Geometry: final body of the model. Coordinates: model frame, mm. Face numbers are marked on the shaded views. A direction names the side the tool comes from. Give positions to 0.01 mm unless a question says otherwise; leave off trailing zeros. Order: outer loops, then holes, each group sorted by start corner. A loop starts at its lowest first (then second) coordinate and runs counter-clockwise, first axis right, second up. Notation, with made-up numbers: (57, -13) - (112, -13) arc R29 ccw to (112, 11) - close; hole circle Ø6 at (62, -8). An arc over 180 degrees is marked (long way). Put each result on its own line as item: value. Start each with the question number.
1. Section B-B on x = -45. Return the cut outline in (y, z).
2. Section D-D on y = 6.25. Return the cut outline in (x, z).
3. Ray query, line 1 along X through (y, z) = (16.5, 3); line 2 along Z through (x, y) = (-31.5, 14.75); line 3 along X through (y, z) = (3, 25). Return the intervals inside material, ascending. Write a range as from..to.
4. First-contact query: P1, Ø15, axis at x = -91.313, y = 14.351, coming from the +Z side. Flat tip, straight axial feed; report the tip coordinate or a pass-through.
5. Set-up query: the marked faces 1 and 2. Return all of +Z, -Z, +X, -X, +Y, -Y with unobstructed straight access to the full face (end or side cutting, diameter ignored); none if empty.
6. Section C-C on y = 18. Return the cut outline in (x, z).
7. Mould query, pull axis Z, two halves, no side actions, for the marked faces 3, 4, 5 and 6. Classes: pulls with the +Z half, pulls with the -Z half, needs draft (parallel to the pull), parting line crosses it, or undercut.
8. Section A-A on z = 23.5. Return the cut outline in (x, y).
from build123d import *

# Parameters (mm, degrees)
EXTRUDE1_DEPTH = 28.702
SKETCH2_R      = 11.303
EXTRUDE2_DEPTH = 93.609737566
SKETCH3_R      = 6.35
EXTRUDE3_DEPTH = 12.7
SKETCH4_R      = 4.7625
EXTRUDE4_DEPTH = 117.756868277


with BuildPart() as part:
    # Sketch1 → Extrude1 (new body)
    with BuildSketch(Plane(origin=(0, 0, 0), x_dir=(1, 0, 0), z_dir=(0, 1, 0))):
        Polygon((0, 0), (0, -35.052), (-28.702, -35.052), (-28.702, -6.35), (-109.474, -6.35), (-109.474, 0), align=None)
    extrude(amount=EXTRUDE1_DEPTH)

    # Sketch2 → Extrude2 (cut, through all)
    with BuildSketch(Plane.ZY.offset(28.702)):
        with Locations((20.701, 14.351)):
            Circle(SKETCH2_R)
    extrude(amount=-EXTRUDE2_DEPTH, mode=Mode.SUBTRACT)

    # Sketch3 → Extrude3 (cut)
    with BuildSketch(Plane.XY.offset(35.052)):
        with Locations((-14.351, 14.351)):
            Circle(SKETCH3_R)
    extrude(amount=-EXTRUDE3_DEPTH, mode=Mode.SUBTRACT)

    # Sketch4 → Extrude4 (cut, through all)
    with BuildSketch(Plane.XY.offset(6.35)):
        with Locations((-91.313, 14.351)):
            Circle(SKETCH4_R)
        with Locations(Location((-46.863, 14.351, 0), (0, 0, 180))):
            Circle(SKETCH4_R)
    extrude(amount=-EXTRUDE4_DEPTH, mode=Mode.SUBTRACT)


solid = part.part
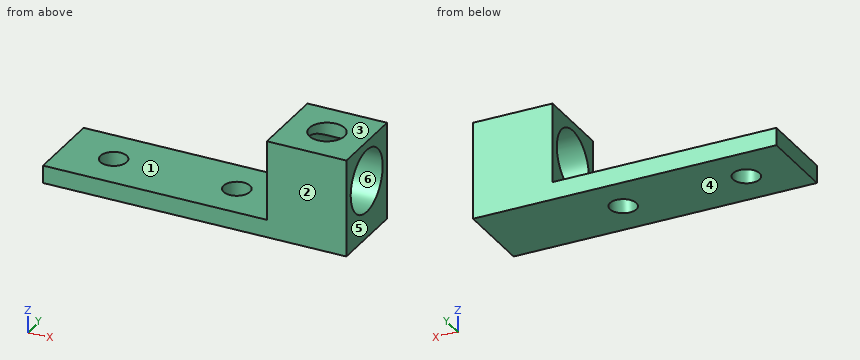
Resolved:
1. outline: (0, 0) - (9.97, 0) - (9.97, 6.35) - (0, 6.35) - close; (18.73, 0) - (28.7, 0) - (28.7, 6.35) - (18.73, 6.35) - close
2. outline: (-109.47, 0) - (0, 0) - (0, 12.82) - (-28.7, 12.82) - (-28.7, 6.35) - (-109.47, 6.35) - close; (-28.7, 28.58) - (0, 28.58) - (0, 35.05) - (-28.7, 35.05) - close
3. line 1: -109.47..-95.56, -87.06..-51.11, -42.61..0
3. line 2: 0..6.35
3. line 3: -28.7..0
4. P1: z = 6.35
5. face 1: +Z, -X, +Y, -Y
5. face 2: +Z, -Z, +X, -X, -Y
6. outline: (-109.47, 0) - (-94.37, 0) - (-94.37, 6.35) - (-109.47, 6.35) - close; (-88.25, 0) - (-49.92, 0) - (-49.92, 6.35) - (-88.25, 6.35) - close; (-43.8, 0) - (0, 0) - (0, 10) - (-28.7, 10) - (-28.7, 6.35) - (-43.8, 6.35) - close; (-28.7, 31.4) - (-19.55, 31.4) - (-19.55, 35.05) - (-28.7, 35.05) - close; (-9.15, 31.4) - (0, 31.4) - (0, 35.05) - (-9.15, 35.05) - close
7. face 3: pulls with the +Z half
7. face 4: pulls with the -Z half
7. face 5: needs draft
7. face 6: undercut
8. outline: (-28.7, 0) - (0, 0) - (0, 3.4) - (-28.7, 3.4) - close; (-28.7, 25.3) - (0, 25.3) - (0, 28.7) - (-28.7, 28.7) - close
